Can you work these out from the drawing? Everything is in mm from the part's minimum corner. Round coordinates to 2 decimals unless told otherwise and drop trailing zeros. Loops run counter-clockwise (first coordinate to the right, second up) from the corner with the lowest first, then second, coordinate; pieces in that order, holes last. Notation, with made-up numbers: M 22.25,81.25 L 70.25,81.25 A15 ccw 70.25,101.25 Z; hole C 88.5,-12 d6. An arc over 180 degrees is marked long. Use a Markdown table: item, result.
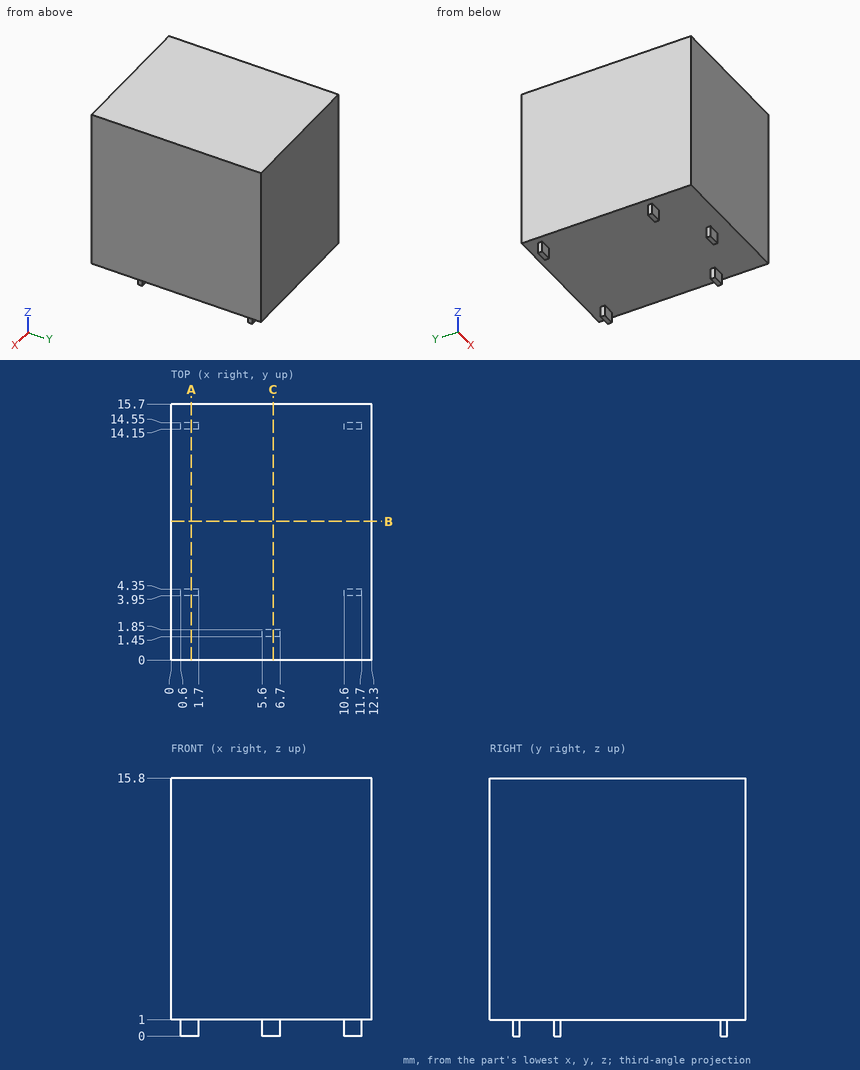
1. I need wall thicknesses on probe 1 along Z at (x, y) = (2.25, 8.75). Which ranges of the line are inside material? Lowest first, please. Write a range as from..to.
Answer sheet:
| item | result |
|---|---|
| probe 1 | 1..15.8 |
2. Imagine slicing it at B-B, the plane y = 8.5. Write out the boundary of the cut face in (x, z), then the cut area to 3 significant figures.
Answer sheet:
| item | result |
|---|---|
| outline | M 0,1 L 12.3,1 L 12.3,15.8 L 0,15.8 Z |
| area | 182 mm2 |
3. Imagine slicing it at A-A, the plane x = 1.25. Write out the boundary of the cut face in (y, z).
Answer sheet:
| item | result |
|---|---|
| outline | M 0,1 L 3.95,1 L 3.95,0 L 4.35,0 L 4.35,1 L 14.15,1 L 14.15,0 L 14.55,0 L 14.55,1 L 15.7,1 L 15.7,15.8 L 0,15.8 Z |
4. Imagine slicing it at C-C, the plane x = 6.25. Write out the boundary of the cut face in (y, z), then the cut area to 3 significant figures.
Answer sheet:
| item | result |
|---|---|
| outline | M 0,1 L 1.45,1 L 1.45,0 L 1.85,0 L 1.85,1 L 15.7,1 L 15.7,15.8 L 0,15.8 Z |
| area | 233 mm2 |
5. For pin 1 Ø0.8 at (x, z) = (6, 0.5) entering from -Y; pin 2 Ø0.5 at (x, z) = (11, 0.5) entering from +Y; pin 3 Ø0.8 at (x, z) = (11.5, 0.5) entering from -Y, each with a flat end and sliding along its axis, tell me the tip position at first contact or that it passes through.
Answer sheet:
| item | result |
|---|---|
| pin 1 | y = 1.45 |
| pin 2 | y = 14.55 |
| pin 3 | y = 3.95 |
